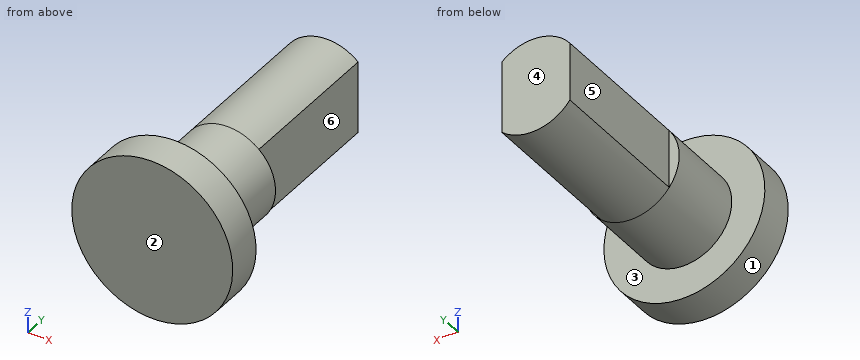
from build123d import *

# Parameters (mm, degrees)
SKETCH1_R           = 4.5
BOSS_EXTRUDE1_DEPTH = 2
SKETCH2_R           = 2.65
BOSS_EXTRUDE2_DEPTH = 4.5
BOSS_EXTRUDE3_DEPTH = 8.5


with BuildPart() as part:
    # Sketch1 → Boss-Extrude1 (new body)
    with BuildSketch(Plane(origin=(0, 0, 0), x_dir=(1, 0, 0), z_dir=(0, 1, 0))):
        with Locations(Location((0, 0, 0), (0, 0, 270))):
            Circle(SKETCH1_R)
    extrude(amount=BOSS_EXTRUDE1_DEPTH)

    # Sketch2 → Boss-Extrude2 (add)
    with BuildSketch(Plane(origin=(0, 2, 0), x_dir=(1, 0, 0), z_dir=(0, 1, 0))):
        with Locations(Location((0, 0, 0), (0, 0, 270))):
            Circle(SKETCH2_R)
    extrude(amount=BOSS_EXTRUDE2_DEPTH)

    # Sketch4 → Boss-Extrude3 (add)
    with BuildSketch(Plane(origin=(0, 6.5, 0), x_dir=(1, 0, 0), z_dir=(0, 1, 0))):
        with BuildLine():
            Line((1.718727688, -2.017046141), (1.718727688, 2.017046141))
            ThreePointArc((1.718727688, 2.017046141), (-0.269470865, 2.63626354), (-2.091272312, 1.627599495))
            Line((-2.091272312, 1.627599495), (-2.091272312, -1.627599495))
            ThreePointArc((-2.091272312, -1.627599495), (-0.269470865, -2.63626354), (1.718727688, -2.017046141))
        make_face()
    extrude(amount=BOSS_EXTRUDE3_DEPTH)


solid = part.part
For this review, take the finished solid that the model builds, in its own axes (mm). Face numbers are marked on the shaded views. A direction names the side the tool comes from. Round coordinates to 2 decimals unless told otherwise and drop trailing zeros. Write each loop counter-clockwise with the first axis right and the second up, starting at its lowest first coordinate (ties: lowest second). Pieces come first, ordered by that corner, then holes. Notation, with made-up numbers: M -1,-15 L 35,-15 A18 cw 35,0 Z; hole C -30.75,30.25 d4. An arc over 180 degrees is marked long. Write item = value, one per line. Start each with the question number.
(1) The part is to be moulded in two halves that separate along Y. For the marked faces 1, 2 and 3, say which applies: +Y half, -Y half, draft (parallel to the pull), parting line (faces both ways), or undercut.
(2) We need section D-D (x = -2.25). Give the boundary of the cut face in (y, z), then the cut area to 3 significant figures.
(3) For the marked faces 4, 5 and 6, list the 3-axis set-ups (+Z, -Z, +X, -X, +Y, -Y) from which the entire face can be reached by the end or side of a thin tool; tool diameter is ignored.
(4) We need section C-C (y = 14.25). Give the boundary of the cut face in (x, z).
(5) We need section A-A (x = 0). Give the boundary of the cut face in (y, z), then the cut area to 3 significant figures.
(6) We need section B-B (z = 0). Give the boundary of the cut face in (x, y).
(7) For line 1 along Y through (x, z) = (3.5, -2.75); line 2 along X through (y, z) = (10.5, -1); line 3 along Y through (x, z) = (2, 0.25), list the stretches that pass through material, from the lowest coordinate up.
(8) Clearance check with flat-ended pins moving along their axes: pin 1 Ø3 at (y, z) = (7.5, -2.5) entering from +X; pin 2 Ø2 at (x, y) = (-1.5, 12) entering from -Z; pin 3 Ø2 at (y, z) = (12, 0.5) entering from +X. State where each tip first meets the part, or that it passes through.
Results found:
q1.face_1 = draft
q1.face_2 = -Y half
q1.face_3 = +Y half
q2.outline = M 0,-3.9 L 2,-3.9 L 2,-1.4 L 6.5,-1.4 L 6.5,1.4 L 2,1.4 L 2,3.9 L 0,3.9 Z
q2.area = 28.2 mm²
q3.face_4 = +Z, -Z, +X, -X, +Y
q3.face_5 = +Z, -Z, -X, +Y
q3.face_6 = +Z, -Z, +X, +Y
q4.outline = M -2.09,-1.63 A2.65 ccw 1.72,-2.02 L 1.72,2.02 A2.65 ccw -2.09,1.63 Z
q5.outline = M 0,-4.5 L 2,-4.5 L 2,-2.65 L 15,-2.65 L 15,2.65 L 2,2.65 L 2,4.5 L 0,4.5 Z
q5.area = 86.9 mm²
q6.outline = M -4.5,0 L 4.5,0 L 4.5,2 L 2.65,2 L 2.65,6.5 L 1.72,6.5 L 1.72,15 L -2.09,15 L -2.09,6.5 L -2.65,6.5 L -2.65,2 L -4.5,2 Z
q7.line_1 = 0 to 2
q7.line_2 = -2.09 to 1.72
q7.line_3 = 0 to 6.5
q8.pin_1 = 2.26
q8.pin_2 = -2.6
q8.pin_3 = 1.72
